Can you work these out from the model? Positions are in its coordinate system, mm. A direction names the side the tool comes from. Give positions to 0.01 mm unless a question says otherwise; leave off trailing zeros. Write each loop counter-clockwise with the first axis right and the second up, starting at its lowest first coordinate (ties: lowest second). Pieces come first, ordered by that corner, then holes.
1. Suppose I cut it at A-A (y = 0). Please give me the cut outline in (x, z).
2. Thinking about a two-plate mould opening in Z: for faces 1 (the cylindrical face through (-2.1, 0, -24.8)), 2 (the flat face through (-1, 0, 25.5)), 3 (the flat face through (0, 0, -20)), which applies, pulls with the +Z half, pulls with the -Z half, needs draft (parallel to the pull), parting line crosses it, or undercut?
3. If I drill on probe 1 along X at (y, z) = (-0.05, 9); probe 2 along Z at (x, y) = (0.1, -0.05); probe 3 along Y at (x, z) = (0.6, 10.5), over which ranges is the centre line in solid material (lowest first)?
4. On a 3-axis mill with a long thin cutter (end or side, diameter ignored), from which of +Z, -Z, +X, -X, +Y, -Y can I reach the whole of each face in a straight line? I mean faces 4 (the flat face through (0.4, 0, -23)), 5 (the cylindrical face through (2.1, 0, 24.8)), 6 (the flat face through (0.4, 0, 23)). Say none if no direction works.
5. I'm going to push a flat-ended pin straight in: pin 1 (1.2 mm diameter, centred on y = -0.5, z = -23.5, fed in from -X). Where does the tip first touch, or does it pass through?
6. Suppose I cut it at B-B (z = 1). Please give me the cut outline in (x, y).
```python
from build123d import *

# Parameters (mm, degrees)
SKETCH_1_R          = 2
EXTRUDE_1_DEPTH     = 25.5
SKETCH_2_R          = 2.1
EXTRUDE_2_DEPTH     = 1.2
CHAMFER_1_SIZE      = 0.2
SKETCH_3_W          = 0.8
SKETCH_3_H          = 4.5
CUT_EXTRUDE_1_DEPTH = 5.5


# Read off the part's stored shape, not the designer's step: 镜向1
with BuildPart() as part:
    # 草图1 → 凸台-拉伸1 (new body)
    with BuildSketch(Plane.XY):
        Circle(SKETCH_1_R)
    extrude(amount=EXTRUDE_1_DEPTH)

    # 草图2 → 凸台-拉伸2 (add)
    with BuildSketch(Plane.XY.offset(25.5)):
        Circle(SKETCH_2_R)
    extrude(amount=-EXTRUDE_2_DEPTH)

    # 倒角1
    chamfer_1_edges = [part.edges().sort_by_distance(p)[0] for p in [
        (-2.1, 0, 25.5),
    ]]
    chamfer(chamfer_1_edges, length=CHAMFER_1_SIZE)

    # 草图3 → 切除-拉伸1 (cut)
    with BuildSketch(Plane.XY.offset(25.5)):
        Rectangle(SKETCH_3_W, SKETCH_3_H)
    extrude(amount=-CUT_EXTRUDE_1_DEPTH, mode=Mode.SUBTRACT)

    # 镜向1: part across plane


with BuildPart() as part_1:
    add(part.part)
    add(part.part.mirror(Plane.XY))


solid = part_1.part
```
Checks:
1. outline: (-2.1, -25.3) - (-1.9, -25.5) - (-0.4, -25.5) - (-0.4, -20) - (0.4, -20) - (0.4, -25.5) - (1.9, -25.5) - (2.1, -25.3) - (2.1, -24.3) - (2, -24.3) - (2, 24.3) - (2.1, 24.3) - (2.1, 25.3) - (1.9, 25.5) - (0.4, 25.5) - (0.4, 20) - (-0.4, 20) - (-0.4, 25.5) - (-1.9, 25.5) - (-2.1, 25.3) - (-2.1, 24.3) - (-2, 24.3) - (-2, -24.3) - (-2.1, -24.3) - close
2. face 1: needs draft
2. face 2: pulls with the +Z half
2. face 3: pulls with the -Z half
3. probe 1: x = -2 to 2
3. probe 2: z = -20 to 20
3. probe 3: y = -1.91 to 1.91
4. face 4: -Z, +Y, -Y
4. face 5: +Z, -Z, +X
4. face 6: +Z, +Y, -Y
5. pin 1: stops at x = -2
6. outline: circle Ø4 at (0, 0)
